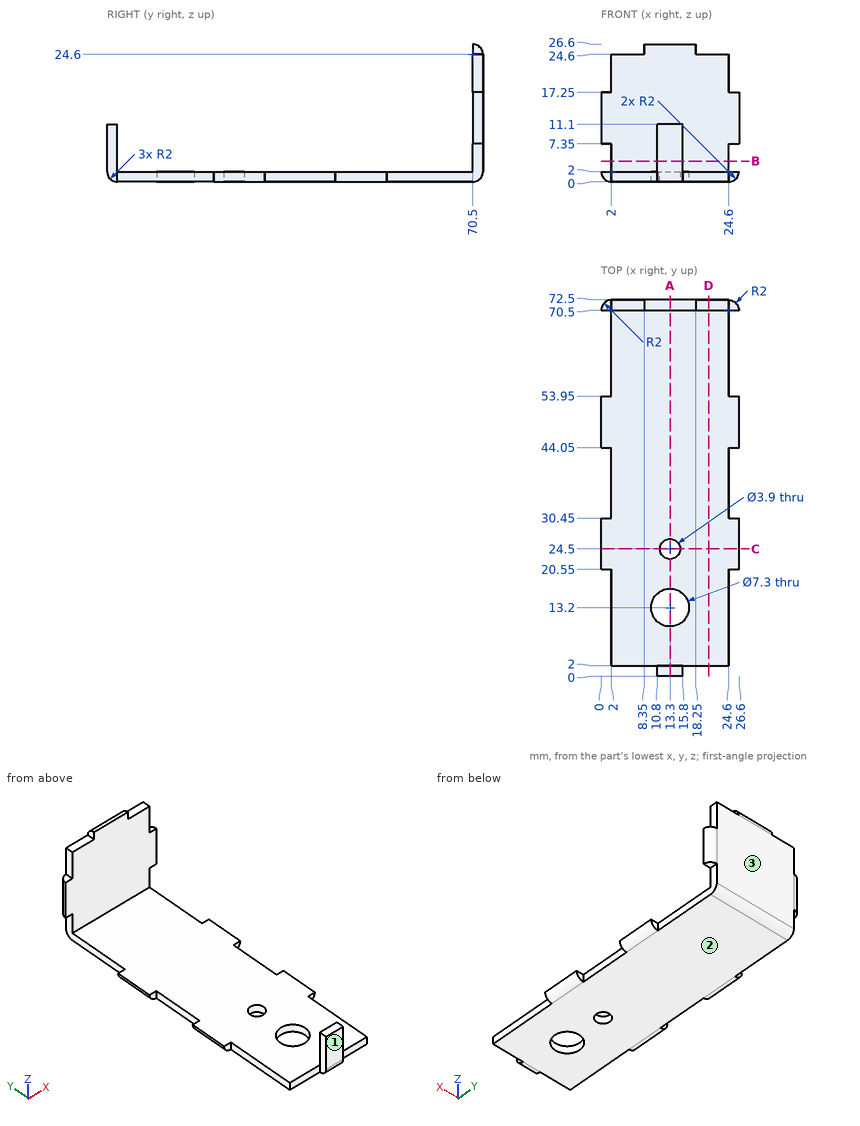
The figure shows three views and two pictorial views of one solid part (mm, origin at its lowest corner). Answer the questions. Round coordinates to 2 decimals unless told otherwise and drop trailing zeros. Order: outer loops, then holes, each group sorted by start corner. A loop starts at its lowest first (then second) coordinate and runs counter-clockwise, first axis right, second up.
Q1. The mould has two halves that part along Y. Classify the marked faces 1, 2 and 3: pulls with the +Y half, pulls with the -Y half, needs draft (parallel to the pull), parting line crosses it, or undercut.
Solution:
face 1: pulls with the -Y half
face 2: needs draft
face 3: pulls with the +Y half
Q2. A cutting plane is placed at D-D, the plane x = 20.75. Determine the outline of the cut face in (y, z), then the cut area to 3 significant figures.
Solution:
outline: (2, 0) - (70.5, 0) arc R2 ccw to (72.5, 2) - (72.5, 24.6) - (70.5, 24.6) - (70.5, 2) - (2, 2) - close
area: 185 mm2
Q3. Given pin 1 Ø0.6 at (x, z) = (20, 0.5) entering from -Y; pin 2 Ø1.5 at (y, z) = (27, 4.5) entering from +X; pin 3 Ø0.6 at (x, z) = (25.5, 1) entering from +Y; pin 4 Ø4 at (x, y) = (4, 53) entering from +Z, each flat-ended and moving along its own axis, determine where each tip first touches the part or whether it passes through.
Solution:
pin 1: stops at y = 2
pin 2: passes through
pin 3: stops at y = 53.95
pin 4: stops at z = 2
Q4. A cutting plane is placed at C-C, the plane y = 24.5. Determine the outline of the cut face in (x, z), then the cut area to 3 significant figures.
Solution:
outline: (0, 2) arc R2 ccw to (2, 0) - (11.35, 0) - (11.35, 2) - close; (15.25, 0) - (24.6, 0) arc R2 ccw to (26.6, 2) - (15.25, 2) - close
area: 43.7 mm2
Q5. A cutting plane is placed at A-A, the plane x = 13.3. Determine the outline of the cut face in (y, z), then the cut area to 3 significant figures.
Solution:
outline: (0, 2) arc R2 ccw to (2, 0) - (9.55, 0) - (9.55, 2) - (2, 2) - (2, 11.1) - (0, 11.1) - close; (16.85, 0) - (22.55, 0) - (22.55, 2) - (16.85, 2) - close; (26.45, 0) - (70.5, 0) arc R2 ccw to (72.5, 2) - (72.5, 24.6) arc R2 ccw to (70.5, 26.6) - (70.5, 2) - (26.45, 2) - close
area: 187 mm2
Q6. Find the intervals of material crossed by line 1 along Y through (x, z) = (13.3, 0.75); line 2 along Z through (x, y) = (2.5, 5); line 3 along Y through (x, z) = (3.75, 22.5), in increasing order.
Solution:
line 1: y = 0.44 to 9.55, 16.85 to 22.55, 26.45 to 72.06
line 2: z = 0 to 2
line 3: y = 70.5 to 72.5
Q7. A cutting plane is placed at B-B, the plane z = 4. Determine the outline of the cut face in (x, y).
Solution:
outline: (2, 70.5) - (24.6, 70.5) - (24.6, 72.5) - (2, 72.5) - close; (10.8, 0) - (15.8, 0) - (15.8, 2) - (10.8, 2) - close
